Can you work these out from the model? Positions are in its coordinate system, mm. A direction names the side the tool comes from. Give positions to 0.01 mm unless a question says otherwise; leave off trailing zeros. Order: outer loops, then holes, each group sorted by start corner. A loop starts at its lowest first (then second) coordinate and runs counter-clockwise, first axis right, second up. Notation, with made-up numbers: M 79.5,44.25 L 102.5,44.25 A26 ccw 102.5,78.25 Z; hole C -35,-4.75 d1. An arc over 180 degrees is marked long. Use a Markdown table: item, result. Add a question column.
from build123d import *

# Parameters (mm, degrees)
F2_DEPTH  = 1.016
F1_W      = 465.328
F1_H      = 309.88
F3_DEPTH  = 2.54
F4_W      = 9.144
F4_H      = 7.112
F4_R      = 3.244327
F4_R_2    = 2.929592
F4_R_3    = 3.265372
F4_W_2    = 19.05
F4_H_2    = 5.08
F4_R_4    = 2.560914
F4_R_5    = 2.816864
F4_R_6    = 5.08
F5_DEPTH  = 25.4
F6_R      = 3.175
F6_R_2    = 3.08912
F7_DEPTH  = 25.4
F8_R      = 3.01306
F8_R_2    = 3.150036
F8_R_3    = 3.123892
F8_R_4    = 2.562744
F8_R_5    = 2.562742
F8_R_6    = 2.755693
F8_R_7    = 2.77302
F8_R_8    = 2.574682
F8_R_9    = 2.625675
F9_DEPTH  = 25.4
F11_DEPTH = 25.4
F13_DEPTH = 25.4


with BuildPart() as f2:
    # F0 (on Front) → F2 (new body)
    with BuildSketch(Plane.XZ):
        with BuildLine():
            ThreePointArc((246.888, 191.262), (241.308384, 204.732384), (227.838, 210.312))
            Line((227.838, 210.312), (-227.838, 210.312))
            ThreePointArc((-227.838, 210.312), (-241.308384, 204.732384), (-246.888, 191.262))
            Line((-246.888, 191.262), (-246.888, -191.262))
            ThreePointArc((-246.888, -191.262), (-241.308384, -204.732384), (-227.838, -210.312))
            Line((-227.838, -210.312), (227.838, -210.312))
            ThreePointArc((227.838, -210.312), (241.308384, -204.732384), (246.888, -191.262))
            Line((246.888, -191.262), (246.888, 191.262))
        make_face()
    extrude(amount=F2_DEPTH)

    # F1 (on Front) → F3 (cut)
    with BuildSketch(Plane.XZ):
        with Locations((0, 41.148)):
            Rectangle(F1_W, F1_H)
    extrude(amount=F3_DEPTH, mode=Mode.SUBTRACT)

    # F4 (on Front) → F5 (cut)
    with BuildSketch(Plane.XZ):
        with Locations((0.508, 201.676)):
            Rectangle(F4_W, F4_H)
        with Locations((-13.079926, 201.966628)):
            Circle(F4_R)
        with Locations((9.968346, 202.251166)):
            Circle(F4_R_2)
        with Locations((18.50475, 201.966628)):
            Circle(F4_R_3)
        with Locations((46.355, 202.692)):
            Rectangle(F4_W_2, F4_H_2)
        with Locations((68.58, 202.692)):
            Circle(F4_R_4)
        with Locations((203.708, 202.692)):
            Circle(F4_R_5)
        with Locations((0, -120.904)):
            Circle(F4_R_6)
    extrude(amount=F5_DEPTH, mode=Mode.SUBTRACT)

    # F6 (on Front) → F7 (cut)
    with BuildSketch(Plane.XZ):
        with Locations((60.96, 202.376222)):
            Circle(F6_R)
        with Locations((-69.582123, 203.2)):
            Circle(F6_R)
        with Locations((-85.958709, 203.2)):
            Circle(F6_R)
        with Locations((-206.248, 203.2)):
            Circle(F6_R)
        with Locations((104.648, -119.617626)):
            Circle(F6_R_2)
    extrude(amount=F7_DEPTH, mode=Mode.SUBTRACT)

    # F8 (on Front) → F9 (cut)
    with BuildSketch(Plane.XZ):
        with Locations((-183.388, -120.360881)):
            Circle(F8_R)
        with Locations((-80.264, -119.844757)):
            Circle(F8_R_2)
        with Locations((182.88, -120.142)):
            Circle(F8_R_3)
        with Locations((-238.76, 147.828)):
            Circle(F8_R_4)
        with Locations((-238.76, 46.228)):
            Circle(F8_R_5)
        with Locations((-238.76, -48.768)):
            Circle(F8_R_6)
        with Locations((238.76, 121.412)):
            Circle(F8_R_7)
        with Locations((238.76, 45.212)):
            Circle(F8_R_8)
        with Locations((238.76, -36.068)):
            Circle(F8_R_9)
    extrude(amount=F9_DEPTH, mode=Mode.SUBTRACT)

    # F10 (on Front) → F11 (cut)
    with BuildSketch(Plane.XZ):
        Polygon((-232.744792, -134.087231), (-239.094792, -134.087231), (-169.244792, -203.937231), (-162.894792, -203.937231), align=None)
        Polygon((-213.694792, -134.087231), (-220.044792, -134.087231), (-169.244792, -184.887231), (-162.894792, -184.887231), align=None)
        Polygon((-232.744792, -152.720597), (-239.094792, -152.720597), (-187.878158, -203.937231), (-181.528158, -203.937231), align=None)
        Polygon((-232.744792, -169.58518), (-239.094792, -169.58518), (-204.742741, -203.937231), (-198.392741, -203.937231), align=None)
        Polygon((-232.744792, -185.633731), (-239.094792, -185.633731), (-220.791292, -203.937231), (-214.441292, -203.937231), align=None)
        Polygon((-169.244792, -168.497142), (-162.894792, -168.497142), (-197.304703, -134.087231), (-203.654703, -134.087231), align=None)
        Polygon((-169.244792, -151.360553), (-162.894792, -151.360553), (-180.168115, -134.087231), (-186.518115, -134.087231), align=None)
        Polygon((165.107568, -203.937231), (171.457568, -203.937231), (241.307568, -134.087231), (234.957568, -134.087231), align=None)
        Polygon((216.654067, -203.937231), (223.004067, -203.937231), (241.307568, -185.633731), (234.957568, -185.633731), align=None)
        Polygon((200.605517, -203.937231), (206.955517, -203.937231), (241.307568, -169.58518), (234.957568, -169.58518), align=None)
        Polygon((183.740934, -203.937231), (190.090934, -203.937231), (241.307568, -152.720597), (234.957568, -152.720597), align=None)
        Polygon((165.107568, -184.887231), (171.457568, -184.887231), (222.257568, -134.087231), (215.907568, -134.087231), align=None)
        Polygon((165.107568, -168.497142), (171.457568, -168.497142), (205.867479, -134.087231), (199.517479, -134.087231), align=None)
        Polygon((165.107568, -151.360553), (171.457568, -151.360553), (188.73089, -134.087231), (182.38089, -134.087231), align=None)
    extrude(amount=F11_DEPTH, mode=Mode.SUBTRACT)

    # F12 (on Front) → F13 (cut)
    with BuildSketch(Plane.XZ):
        with BuildLine():
            ThreePointArc((-250.468968, 134.112), (-246.872017, 140.014539), (-245.618, 146.812))
            ThreePointArc((-245.618, 146.812), (-271.465461, 164.607983), (-278.867032, 134.112))
            ThreePointArc((-278.867032, 134.112), (-264.668, 140.462), (-250.468968, 134.112))
        make_face()
        with BuildLine():
            ThreePointArc((-250.468968, 134.112), (-264.668, 127.762), (-278.867032, 134.112))
            ThreePointArc((-278.867032, 134.112), (-283.718, 121.412), (-278.867032, 108.712))
            ThreePointArc((-278.867032, 108.712), (-264.668, 115.062), (-250.468968, 108.712))
            ThreePointArc((-250.468968, 108.712), (-246.872017, 114.614539), (-245.618, 121.412))
            ThreePointArc((-245.618, 121.412), (-246.872017, 128.209461), (-250.468968, 134.112))
        make_face()
        with BuildLine():
            ThreePointArc((-250.468968, 108.712), (-264.668, 102.362), (-278.867032, 108.712))
            ThreePointArc((-278.867032, 108.712), (-271.465461, 78.216017), (-245.618, 96.012))
            ThreePointArc((-245.618, 96.012), (-246.872017, 102.809461), (-250.468968, 108.712))
        make_face()
        with BuildLine():
            ThreePointArc((278.867032, 134.112), (282.463983, 140.014539), (283.718, 146.812))
            ThreePointArc((283.718, 146.812), (257.870539, 164.607983), (250.468968, 134.112))
            ThreePointArc((250.468968, 134.112), (264.668, 140.462), (278.867032, 134.112))
        make_face()
        with BuildLine():
            ThreePointArc((278.867032, 134.112), (264.668, 127.762), (250.468968, 134.112))
            ThreePointArc((250.468968, 134.112), (245.618, 121.412), (250.468968, 108.712))
            ThreePointArc((250.468968, 108.712), (264.668, 115.062), (278.867032, 108.712))
            ThreePointArc((278.867032, 108.712), (282.463983, 114.614539), (283.718, 121.412))
            ThreePointArc((283.718, 121.412), (282.463983, 128.209461), (278.867032, 134.112))
        make_face()
        with BuildLine():
            ThreePointArc((278.867032, 108.712), (264.668, 102.362), (250.468968, 108.712))
            ThreePointArc((250.468968, 108.712), (257.870539, 78.216017), (283.718, 96.012))
            ThreePointArc((283.718, 96.012), (282.463983, 102.809461), (278.867032, 108.712))
        make_face()
    extrude(amount=F13_DEPTH, mode=Mode.SUBTRACT)


solid = f2.part
1. If we section it at B-B, the plane x = -128: List the corners of the cut face in (y, z) for me, then the cut area to 3 significant figures.
2. We'd pull the mould along X, two halves only. Please class faces 1 (the face through (241.16, -0.5, -204.88)), 2 (the face through (-178.002, -0.501, -142.603)), 3 (the face through (17, -1.016, -124)): +X half, -X half, draft (parallel to the pull), parting line (faces both ways), or undercut.
3. On a 3-axis mill with a long thin cutter (end or side, diameter ignored), from which of +Z, -Z, +X, -X, +Y, -Y can I reach the whole of each face in a straight line? I mean faces 4 (the face through (-241.46, -0.5, -204.58)), 5 (the face through (182.553, -0.501, -151.051)). Say none if no direction works.
4. If we section it at A-A, the plane z = 76: List the corners of the cut face in (x, y) for me.
5. If we section it at C-C, the plane y = -0.85: State how many separate pieces and enclosed holes the cut face has, then the cut area to 3 significant figures.
6. I need wall thicknesses on L1, parallel to Z at x = 138.5, y = -0.65; L2, parallel to X at y = -0.8, z = 88.5; L3, parallel to Z at x = 11, y = -0.85. Which ranges of each line are inside material? Lowest first, please. Write a range as [from, to].
Geometry results:
| question | item | result |
|---|---|---|
| 1 | outline | M -1.02,-210.31 L 0,-210.31 L 0,-113.79 L -1.02,-113.79 Z; M -1.02,196.09 L 0,196.09 L 0,210.31 L -1.02,210.31 Z |
| 1 | area | 113 mm^2 |
| 2 | face 1 | +X half |
| 2 | face 2 | undercut |
| 2 | face 3 | draft |
| 3 | face 4 | -Z, -X, +Y, -Y |
| 3 | face 5 | +Y, -Y |
| 4 | outline | M -246.89,-1.02 L -232.66,-1.02 L -232.66,0 L -246.89,0 Z; M 232.66,-1.02 L 246.89,-1.02 L 246.89,0 L 232.66,0 Z |
| 5 | separate pieces | 1 |
| 5 | enclosed holes | 37 |
| 5 | area | 58,800 mm^2 |
| 6 | L1 | z = [-210.31, -113.79], [196.09, 210.31] |
| 6 | L2 | x = [-246.89, -232.66], [232.66, 246.89] |
| 6 | L3 | z = [-210.31, -113.79], [196.09, 199.51], [204.99, 210.31] |
